```python
from build123d import *

# Parameters (mm, degrees)
SKETCH1_R           = 15
SKETCH1_R_2         = 13.5
BOSS_EXTRUDE1_DEPTH = 80
SKETCH2_R           = 3
CUT_EXTRUDE1_DEPTH  = 33
SKETCH3_R           = 3
CUT_EXTRUDE2_DEPTH  = 33


with BuildPart() as part:
    # Sketch1 → Boss-Extrude1 (new body)
    with BuildSketch(Plane.XY):
        Circle(SKETCH1_R)
        Circle(SKETCH1_R_2, mode=Mode.SUBTRACT)
    extrude(amount=BOSS_EXTRUDE1_DEPTH)

    # Sketch2 → Cut-Extrude1 (cut, symmetric)
    with BuildSketch(Plane(origin=(0, 0, 0), x_dir=(1, 0, 0), z_dir=(0, 1, 0))):
        with Locations(Location((0, -5, 0), (0, 0, 270))):
            Circle(SKETCH2_R)
    extrude(amount=CUT_EXTRUDE1_DEPTH, both=True, mode=Mode.SUBTRACT)

    # Sketch3 → Cut-Extrude2 (cut, symmetric)
    with BuildSketch(Plane.XZ):
        with Locations(Location((0, 71.839569, 0), (0, 0, 270))):
            Circle(SKETCH3_R)
    extrude(amount=CUT_EXTRUDE2_DEPTH, both=True, mode=Mode.SUBTRACT)


solid = part.part
```
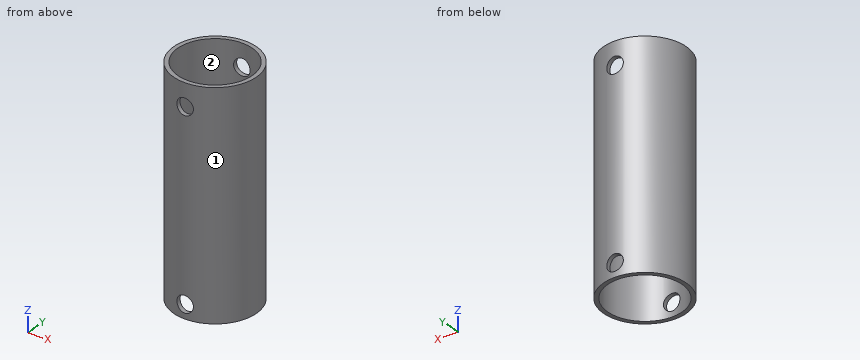
For this review, take the finished solid that the model builds, in its own axes (mm). Face numbers are marked on the shaded views. Round coordinates to 2 decimals unless told otherwise and drop trailing zeros. Write each loop counter-clockwise with the first axis right and the second up, starting at its lowest first coordinate (ties: lowest second). Pieces come first, ordered by that corner, then holes. Notation, with made-up numbers: (81, -15) - (100, -15) arc R29 cw to (100, 6) - close; hole circle Ø1 at (-4.5, 7.25). An arc over 180 degrees is marked (long way). Answer as CSV lines item,"result". Start each with the question number.
(1) Add section D-D, the plane z = 56. State the section outline as (x, y) points.
(2) Mouldability with a two-part tool opening along Y and no side actions: class the marked faces 1 and 2 as +Y half, -Y half, draft (parallel to the pull), parting line (faces both ways), or undercut.
(3) Add section A-A, the plane x = 0. State the section outline as (y, z) points, plus the area to 3 significant figures.
(4) Add section B-B, the plane y = 0. State the section outline as (x, z) points, plus the area to 3 significant figures.
(5) Add section C-C, the plane x = 12. State the section outline as (y, z) points, plus the area to 3 significant figures.
(6) For pin 1 (3.5 mm diameter, centred on x = 0, z = 71.84, fed in from +Y); pin 2 (1 mm diameter, centred on y = -2.5, z = 36, fed in from -X); pin 3 (12 mm diameter, centred on y = -10, z = 45, fed in from -X); pin 4 (1 mm diameter, centred on x = 2.5, z = 58.5, fed in from -Y), all flat-tipped, find the tip position at first contact; note any pin that passes through.
(7) For line 1 (Z direction, x = 0, y = -14); line 2 (Y direction, x = 0, z = 38); line 3 (Y direction, x = -9, z = 35.5), list the stretches that pass through material, from the lowest coordinate up.
From the geometry:
1,outline,"circle Ø30 at (0, 0); hole circle Ø27 at (0, 0)"
2,face 1,"parting line"
2,face 2,"undercut"
3,outline,"(-15, 0) - (-13.5, 0) - (-13.5, 2) - (-15, 2) - close; (-15, 8) - (-13.5, 8) - (-13.5, 68.84) - (-15, 68.84) - close; (-15, 74.84) - (-13.5, 74.84) - (-13.5, 80) - (-15, 80) - close; (13.5, 0) - (15, 0) - (15, 2) - (13.5, 2) - close; (13.5, 8) - (15, 8) - (15, 68.84) - (13.5, 68.84) - close; (13.5, 74.84) - (15, 74.84) - (15, 80) - (13.5, 80) - close"
3,area,"204 mm²"
4,outline,"(-15, 0) - (-13.5, 0) - (-13.5, 80) - (-15, 80) - close; (13.5, 0) - (15, 0) - (15, 80) - (13.5, 80) - close"
4,area,"240 mm²"
5,outline,"(-9, 0) - (-6.18, 0) - (-6.18, 80) - (-9, 80) - close; (6.18, 0) - (9, 0) - (9, 80) - (6.18, 80) - close"
5,area,"450 mm²"
6,pin 1,"passes through"
6,pin 2,"stops at x = -14.87"
6,pin 3,"stops at x = -14.46"
6,pin 4,"stops at y = -14.87"
7,line 1,"z = 0 to 2, 8 to 68.84, 74.84 to 80"
7,line 2,"y = -15 to -13.5, 13.5 to 15"
7,line 3,"y = -12 to -10.06, 10.06 to 12"
